Geometry: final body of the model. Coordinates: model frame, mm. Coordinates: 2 decimals unless noted, no trailing zeros. Order: outer loops, then holes, each group sorted by start corner. A loop starts at its lowest first (then second) coordinate and runs counter-clockwise, first axis right, second up. Notation, with made-up numbers: (-20.5, 17.25) -> (-9.5, 17.25) arc R20 ccw to (-9.5, 26.25) -> close; hole circle Ø10 at (-26, 24.25). An arc over 180 degrees is marked (long way). Use one line per item in the form item = value.
Autodesk Inventor part; units mm, degrees
ref_plane "YZ Plane" through (0, 0, 0) normal (1, 0, 0) x (0, 1, 0)
ref_plane "XZ Plane" through (0, 0, 0) normal (0, 1, 0) x (-1, 0, 0)
ref_plane "XY Plane" through (0, 0, 0) normal (0, 0, 1) x (1, 0, 0)
sketch "Sketch1" plane through (0, 0, 0) normal (0, 1, 0) x (-1, 0, 0)
  circle A0 centre (0, 0) radius 177
  dimension "d0" = 354
extrude "Extrusion1" add sketch "Sketch1" along normal blind 5
sketch "Sketch2" plane through (0, 5, 0) normal (0, 1, 0) x (1, 0, 0)
  circle A0 centre (-114.3, 82.55) radius 1.7
  line L0 (-177, 0) -> (177, 0) construction
  line L1 (0, 177) -> (0, -177) construction
  circle A1 centre (114.3, 82.55) radius 1.7
  circle A2 centre (-114.3, -82.55) radius 1.7
  circle A3 centre (114.3, -82.55) radius 1.7
  point P0 (0, 0)
  dimension "d3" = 3.4
  dimension "d20" = 82.55
  dimension "d21" = 114.3
  dimension "d24" = 228.6
  dimension "d27" = 165.1
extrude "Level2 Standoffs" cut sketch "Sketch2" against normal through all
sketch "Sketch3" plane through (0, 5, 0) normal (0, 1, 0) x (1, 0, 0)
  circle A0 centre (-127, 50.8) radius 10.16
  circle A1 centre (127, 50.8) radius 10.16
  circle A2 centre (0, 0) radius 177 construction
  line L0 (0, 177) -> (0, -177) construction
  line L1 (177, 0) -> (-177, 0) construction
  circle A3 centre (0, 0) radius 177 construction
  dimension "d32" = 20.32
  dimension "d33" = 20.32
  dimension "d34" = 127
  dimension "d35" = 127
  dimension "d36" = 50.8
  dimension "d37" = 50.8
extrude "Wires" cut sketch "Sketch3" against normal through all
sketch "Sketch4" plane through (0, 5, 0) normal (0, 1, 0) x (1, 0, 0)
  line L0 (0, 0) -> (153.2865, -88.5) construction
  circle A0 centre (0, 0) radius 177 construction
  line L1 (-177, 0) -> (177, 0) construction
  circle A1 centre (142.288, -82.15) radius 1.7
  line L2 (142.288, -82.15) -> (134.0391, -77.3875) construction
  line L3 (134.0391, -232.1625) -> (134.0391, -55.1625) construction
  circle A2 centre (134.0391, -67.8625) radius 1.7
  line L4 (268.0782, 0) -> (114.7917, -88.5) construction
  circle A3 centre (125.7902, -82.15) radius 1.7
  circle A4 centre (125.7902, 82.15) radius 1.7
  circle A5 centre (142.288, 82.15) radius 1.7
  circle A6 centre (134.0391, 67.8625) radius 1.7
  line L5 (0, 177) -> (0, -177) construction
  circle A7 centre (-142.288, -82.15) radius 1.7
  circle A8 centre (-134.0391, -67.8625) radius 1.7
  circle A9 centre (-125.7902, -82.15) radius 1.7
  circle A10 centre (-125.7902, 82.15) radius 1.7
  circle A11 centre (-142.288, 82.15) radius 1.7
  circle A12 centre (-134.0391, 67.8625) radius 1.7
  dimension "d40" = 30
  dimension "d41" = 12.7
  dimension "d42" = 9.525
  dimension "d45" = 360
  dimension "d49" = 60
  dimension "d65" = 3.4
extrude "Level4 Standoffs" cut sketch "Sketch4" against normal through all
sketch "Sketch5" plane through (0, 5, 0) normal (0, 1, 0) x (1, 0, 0)
  circle A0 centre (0, -141.44) radius 2.667
  circle A1 centre (0, 0) radius 177 construction
  line L0 (0, -177) -> (89.0082, -177) construction
  circle A2 centre (100.0132, -100.0132) radius 2.667
  circle A3 centre (141.44, 0) radius 2.667
  circle A4 centre (100.0132, 100.0132) radius 2.667
  circle A5 centre (0, 141.44) radius 2.667
  circle A6 centre (-100.0132, 100.0132) radius 2.667
  circle A7 centre (-141.44, 0) radius 2.667
  circle A8 centre (-100.0132, -100.0132) radius 2.667
  dimension "d53" = 5.334
  dimension "d54" = 35.56
  dimension "d57" = 360
extrude "Zip Ties" cut sketch "Sketch5" against normal through all
sketch "Sketch6" plane through (0, 5, 0) normal (0, 1, 0) x (1, 0, 0)
  circle A0 centre (0, -88.9) radius 1.7
  point P0 (0, 0)
  dimension "d61" = 3.4
  dimension "d62" = 88.9
extrude "Extrusion6" cut sketch "Sketch6" against normal blind 25.4
equation "\"d0\" = robot_diameter"
equation "\"d1\" = hardboard_thickness"
equation "\"d3\" = m3_clearance"
equation "\"d24\" = 2 * d21"
equation "\"d27\" = 2 * d20"
equation "\"d33\" = d32"
equation "\"d35\" = d34"
equation "\"d37\" = d36"
equation "\"d65\" = m3_clearance"
equation "\"d61\" = m3_clearance"
equation "\"m3_heat_set_insert\" = 4"
equation "\"m3_clearance\" = 3.4"
equation "\"m3_heat_set_depth\" = 7"
equation "\"robot_diameter\" = 354"
equation "\"hardboard_thickness\" = 5"
equation "\"motor_centerline_height\" = 13"
properties part number "layer3_new"
1) Section B-B, the plane z = -50.8. Output: boundary loops of the cut face in (x, y).
Results found:
outline = (-169.55, 0) -> (-137.16, 0) -> (-137.16, 5) -> (-169.55, 5) -> close; (-116.84, 0) -> (116.84, 0) -> (116.84, 5) -> (-116.84, 5) -> close; (137.16, 0) -> (169.55, 0) -> (169.55, 5) -> (137.16, 5) -> close
2) Section A-A, the plane y = 3.25. Give the number of separate pieces and of enclosed holes in the cut face, and give its area (3 significant figures).
Results found:
separate_pieces = 1
enclosed_holes = 27
area = 97,400 mm2
3) Section C-C, the plane x = 81. Output: boundary loops of the cut face in (y, z), and give its area (3 significant figures).
Results found:
outline = (0, -157.38) -> (5, -157.38) -> (5, 157.38) -> (0, 157.38) -> close
area = 1,570 mm2
4) Material intervals for probe 1 along Z at (x, y) = (0, 2); probe 2 along X at (y, z) = (2.85, -50.8); probe 3 along Z at (x, y) = (141.44, 1.2), sorted ascending. Write a range as from..to.
Results found:
probe_1 = -177..-144.11, -138.77..87.2, 90.6..138.77, 144.11..177
probe_2 = -169.55..-137.16, -116.84..116.84, 137.16..169.55
probe_3 = -106.41..-83.62, -80.68..-2.67, 2.67..80.68, 83.62..106.41
5) Section D-D, the plane z = 46. Output: boundary loops of the cut face in (x, y), and give its area (3 significant figures).
Results found:
outline = (-170.92, 0) -> (170.92, 0) -> (170.92, 5) -> (-170.92, 5) -> close
area = 1,710 mm2
6) Pull-direction query (X, two-part tool) for faces 1 (the cylindrical face through (125.677, 2.535, -60.874)), 2 (the flat face through (2, 0, 2)), 3 (the cylindrical face through (38.37, 2.46, 172.79)); classes: released by +X, released by -X, zero draft, split by the parting line, or undercut.
Results found:
face_1 = undercut
face_2 = zero draft
face_3 = split by the parting line
7) Contact query for flat-ended pins moving along their axis: P1, Ø3, axis at x = 5.5, y = 2.5, coming from the +Z side; P2, Ø8.5, axis at x = -100.01, z = 100.01, coming from the -Y side. Output: stop coordinate, or through.
Results found:
P1 = 176.95
P2 = 0
